Drawing for the job (mm, zero at the part's lowest x, y, z). A direction names the side the tool comes from. Coordinates: 2 decimals unless noted, no trailing zeros. Write each loop counter-clockwise with the first axis right and the second up, starting at its lowest first coordinate (ties: lowest second). Pieces come first, ordered by that corner, then holes. Notation, with made-up numbers: (85, -33) - (142, -33) arc R30 ccw to (142, 1) - close; hole circle Ø7 at (-26, 1). An arc over 180 degrees is marked (long way). Write each question's results on one line, items separated by ' | '.
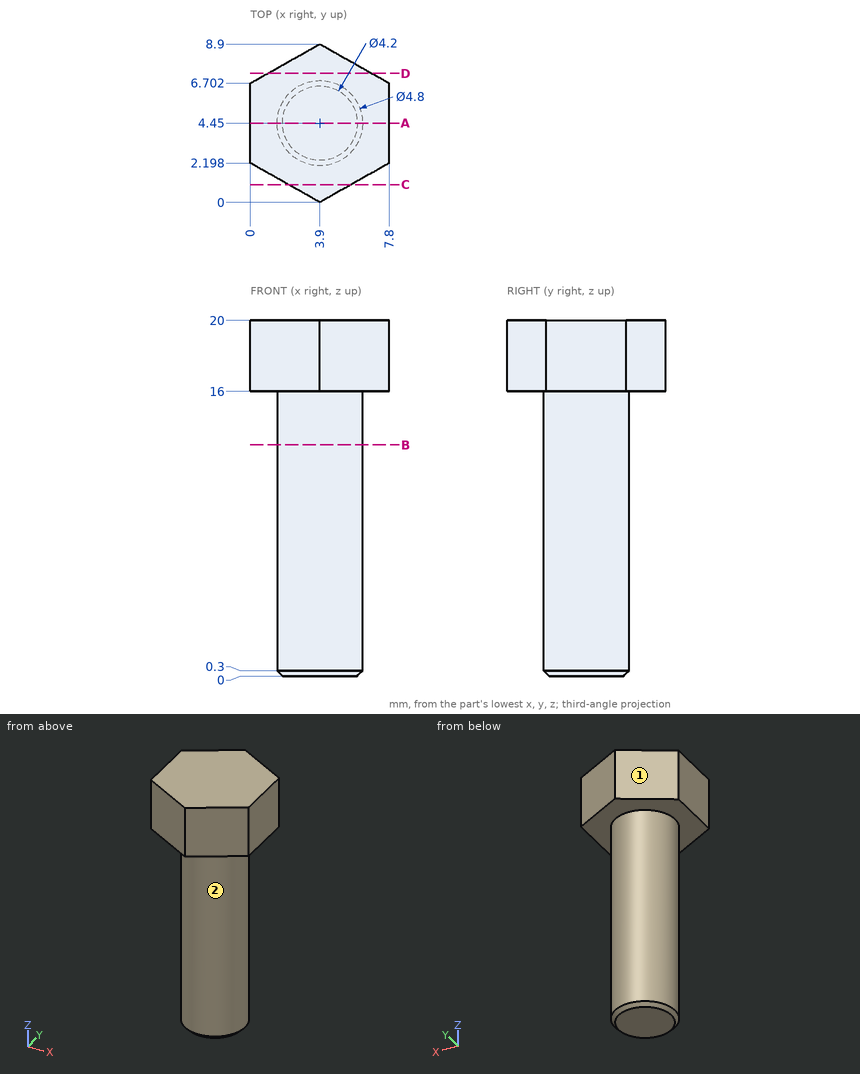
(1) Saw through at D-D on y = 7.25. Write the cut outline in (x, z).
Return value:
outline: (0.97, 16) - (6.83, 16) - (6.83, 20) - (0.97, 20) - close
(2) Saw through at A-A on y = 4.45. Write the cut outline in (x, z), then the cut area to 3 significant figures.
Return value:
outline: (0, 16) - (1.5, 16) - (1.5, 0.3) - (1.8, 0) - (6, 0) - (6.3, 0.3) - (6.3, 16) - (7.8, 16) - (7.8, 20) - (0, 20) - close | area: 108 mm^2
(3) 3-axis set-ups, long thin cutter, end or side, ignore diameter. For the marked faces 1 and 2: which of +Z, -Z, +X, -X, +Y, -Y reach the whole face in a straight line?
Return value:
face 1: +Z, -Z, -X, +Y | face 2: -Z
(4) Saw through at B-B on z = 13. Write the cut outline in (x, y), then the cut area to 3 significant figures.
Return value:
outline: circle Ø4.8 at (3.9, 4.45) | area: 18.1 mm^2
(5) Wall check: line 1 (Z direction, x = 6.5, y = 5.5); line 2 (X direction, y = 2.25, z = 10); line 3 (Y direction, x = 5.75, z = 18.5). Give the ranges that are in metal, low to high. Write a range as from..to.
Return value:
line 1: z = 16..20 | line 2: x = 2.94..4.86 | line 3: y = 1.04..7.86
(6) Saw through at C-C on y = 1. Write the cut outline in (x, z).
Return value:
outline: (2.13, 16) - (5.67, 16) - (5.67, 20) - (2.13, 20) - close
(7) Flat gauge pins, fed straight in: P1, Ø1, axis at x = 5.5, z = 13.5, coming from the -Y side; P2, Ø1, axis at x = 6.5, y = 3.5, coming from the -Z side; P3, Ø1, axis at y = 4, z = 8, coming from the -X side. Where does each tip first touch, or does it go through?
Return value:
P1: stops at y = 2.32 | P2: stops at z = 0.17 | P3: stops at x = 1.5
